Geometry: see drawing. Coordinates: mm, zero at the bounding-box minimum. A direction names the side the tool comes from. Coordinates: 2 decimals unless noted, no trailing zeros. Use one line per item in the form item = value.
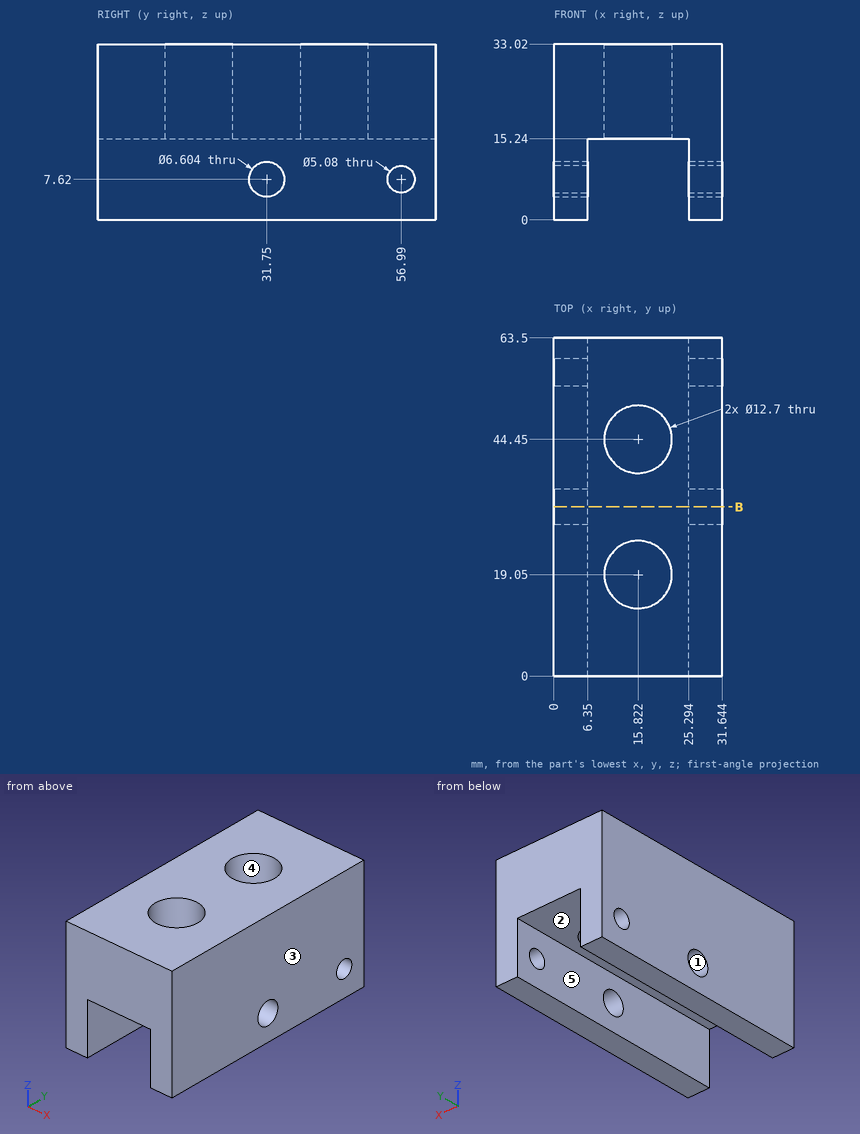
1) Pull-direction query (X, two-part tool) for the marked faces 1, 2 and 3; classes: released by +X, released by -X, zero draft, split by the parting line, or undercut.
Results found:
face_1 = zero draft
face_2 = undercut
face_3 = released by +X
2) Access query for the marked faces 4 and 5. Directions: +Z, -Z, +X, -X, +Y, -Y. A direction counts if a zero-diameter tool reaches every point of the face in a straight line with its end or side. Return the directions, or none.
Results found:
face_4 = +Z, -Z
face_5 = -Z, +Y, -Y
3) Material intervals for probe 1 along Y at (x, z) = (28.25, 7.62); probe 2 along Y at (x, z) = (30, 7); probe 3 along Z at (x, y) = (7.5, 40), sorted ascending. Write a range as from..to.
Results found:
probe_1 = 0..28.45, 35.05..54.45, 59.53..63.5
probe_2 = 0..28.51, 34.99..54.53, 59.45..63.5
probe_3 = 15.24..33.02
4) Section B-B, the plane y = 31.75. Give the number of separate pieces and of enclosed holes in the cut face, and give its area (3 significant figures).
Results found:
separate_pieces = 3
enclosed_holes = 0
area = 672 mm2
